```python
from build123d import *

# Parameters (mm, degrees)
BOSS_EXTRUDE1_DEPTH            = 19.05
F_7_0_201_DIAMETER_HOLE1_D     = 5.1054
F_7_0_201_DIAMETER_HOLE1_DEPTH = 25.4


with BuildPart() as part:
    # Sketch2 → Boss-Extrude1 (new body)
    with BuildSketch(Plane.XY):
        Polygon((0, 47.617699385), (-55.88, 12.7), (-55.88, 0), (0, 0), align=None)
    extrude(amount=BOSS_EXTRUDE1_DEPTH)

    # #7 (0.201) Diameter Hole1
    with Locations(Plane(origin=(-21.399252353, 34.245962436, 0), x_dir=(0.8480480961564308, 0.5299192642331972, 0), z_dir=(-0.5299192642331972, 0.848048096156431, 0))):
        with Locations((-28.741463778, -9.525), (15.708536222, -9.525)):
            Hole(F_7_0_201_DIAMETER_HOLE1_D / 2, depth=F_7_0_201_DIAMETER_HOLE1_DEPTH)


solid = part.part
```
CAD build for the part. Positions are in the model's coordinates, mm. Round coordinates to 2 decimals unless told otherwise and drop trailing zeros. Order: outer loops, then holes, each group sorted by start corner. A loop starts at its lowest first (then second) coordinate and runs counter-clockwise, first axis right, second up.
Q1. Slice it at B-B (x = -16). Write the cut outline in (y, z).
Q2. Two-plate mould, pull along Z, no slides. Class faces 1 (the flat face through (-22, 19, 19.05)), 2 (the cylindrical face through (-37.12, 9.98, 9.41)), 3 (the cylindrical face through (-6.023, 34.831, 10.503)), 4 (the flat face through (0, 23, 9)): pulls with the +Z half, pulls with the -Z half, needs draft (parallel to the pull), parting line crosses it, or undercut.
Q3. Slice it at C-C (z = 4.5). Write the cut outline in (x, y), and give its area (3 significant figures).
Q4. Wall check: L1, parallel to Z at x = -41, y = 9; L2, parallel to X at y = 34.5, z = 8.25; L3, parallel to X at y = 38, z = 10.25. Give the ranges that are in metal, low to high.
Q5. Slice it at A-A (z = 11). Write the cut outline in (x, y).
Q6. Drop flat-ended pins along their axis: pin 1 (5 mm diameter, centred on y = 29, z = 11.5, fed in from -X); pin 2 (5 mm diameter, centred on y = 16, z = 10, fed in from -X); pin 3 (1 mm diameter, centred on x = -34, z = 3.5, fed in from +Y). Give the stop position or say it passes through.
Results below:
1. outline: (0, 0) - (37.62, 0) - (37.62, 19.05) - (0, 19.05) - close
2. face 1: pulls with the +Z half
2. face 2: undercut
2. face 3: undercut
2. face 4: needs draft
3. outline: (-55.88, 0) - (0, 0) - (0, 47.62) - (-55.88, 12.7) - close
3. area: 1,690 mm2
4. L1: z = 0 to 7.3, 11.75 to 19.05
4. L2: x = -20.99 to -5.64, -0.43 to 0
4. L3: x = -15.39 to -8.11, -2.34 to 0
5. outline: (-55.88, 0) - (-36.35, 0) - (-47.54, 17.91) - (-55.88, 12.7) - close; (-44.01, 20.12) - (-31.43, 0) - (0, 0) - (0, 25.71) - (-9.84, 41.47) - close; (-6.31, 43.67) - (0, 33.57) - (0, 47.62) - close
6. pin 1: stops at x = -33.8
6. pin 2: stops at x = -54.6
6. pin 3: stops at y = 26.68
